For this review, take the finished solid that the model builds, in its own axes (mm). Give positions to 0.01 mm unless a question says otherwise; leave off trailing zeros. Order: outer loops, then holes, each group sorted by start corner. A loop starts at its lowest first (then second) coordinate and runs counter-clockwise, first axis right, second up.
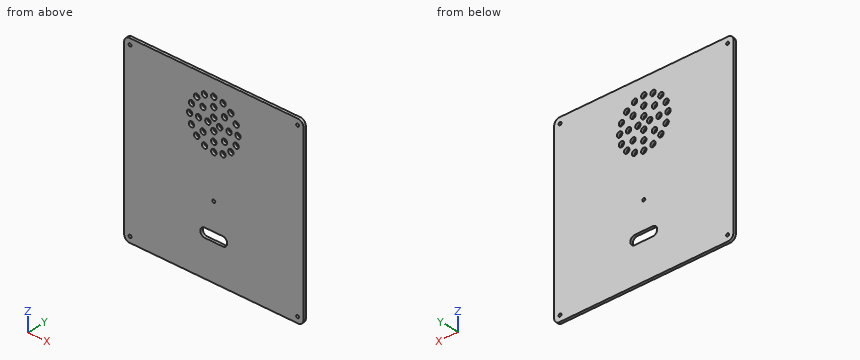
from build123d import *

# Parameters (mm, degrees)
SKETCH1_W           = 200
SKETCH1_H           = 200
SKETCH1_R           = 3
BOSS_EXTRUDE1_DEPTH = 3
FILLET1_R           = 6
FILLET2_R           = 6
FILLET3_R           = 6
FILLET4_R           = 6
SKETCH2_R           = 1.65
SKETCH2_R_2         = 5
CUT_EXTRUDE1_DEPTH  = 283.85862193


with BuildPart() as part:
    # Sketch1 → Boss-Extrude1 (new body)
    with BuildSketch(Plane(origin=(0, 0, 0), x_dir=(1, 0, 0), z_dir=(0, 1, 0))):
        with Locations((100, 100)):
            Rectangle(SKETCH1_W, SKETCH1_H)
        with Locations(Location((116.974857902, 45, 0), (0, 0, 270))):
            Circle(SKETCH1_R, mode=Mode.SUBTRACT)
        with Locations(Location((112.003037132, 32.996962868, 0), (0, 0, 270))):
            Circle(SKETCH1_R, mode=Mode.SUBTRACT)
        with Locations(Location((100, 28.025142098, 0), (0, 0, 270))):
            Circle(SKETCH1_R, mode=Mode.SUBTRACT)
        with Locations(Location((87.996962868, 32.996962868, 0), (0, 0, 270))):
            Circle(SKETCH1_R, mode=Mode.SUBTRACT)
        with Locations(Location((83.025142098, 45, 0), (0, 0, 270))):
            Circle(SKETCH1_R, mode=Mode.SUBTRACT)
        with Locations(Location((87.996962868, 57.003037132, 0), (0, 0, 270))):
            Circle(SKETCH1_R, mode=Mode.SUBTRACT)
        with Locations(Location((100, 61.974857902, 0), (0, 0, 270))):
            Circle(SKETCH1_R, mode=Mode.SUBTRACT)
        with Locations(Location((112.003037132, 57.003037132, 0), (0, 0, 270))):
            Circle(SKETCH1_R, mode=Mode.SUBTRACT)
        with Locations(Location((126.974857902, 45, 0), (0, 0, 270))):
            Circle(SKETCH1_R, mode=Mode.SUBTRACT)
        with Locations(Location((124.921888894, 34.679027829, 0), (0, 0, 270))):
            Circle(SKETCH1_R, mode=Mode.SUBTRACT)
        with Locations(Location((119.075527791, 25.929330111, 0), (0, 0, 270))):
            Circle(SKETCH1_R, mode=Mode.SUBTRACT)
        with Locations(Location((110.325830073, 20.082969008, 0), (0, 0, 270))):
            Circle(SKETCH1_R, mode=Mode.SUBTRACT)
        with Locations(Location((100.004857902, 18.03, 0), (0, 0, 270))):
            Circle(SKETCH1_R, mode=Mode.SUBTRACT)
        with Locations(Location((89.683885731, 20.082969008, 0), (0, 0, 270))):
            Circle(SKETCH1_R, mode=Mode.SUBTRACT)
        with Locations(Location((80.934188014, 25.929330111, 0), (0, 0, 270))):
            Circle(SKETCH1_R, mode=Mode.SUBTRACT)
        with Locations(Location((75.08782691, 34.679027829, 0), (0, 0, 270))):
            Circle(SKETCH1_R, mode=Mode.SUBTRACT)
        with Locations(Location((106.559618743, 45, 0), (0, 0, 270))):
            Circle(SKETCH1_R, mode=Mode.SUBTRACT)
        with Locations(Location((100, 38.440381257, 0), (0, 0, 270))):
            Circle(SKETCH1_R, mode=Mode.SUBTRACT)
        with Locations(Location((93.440381257, 45, 0), (0, 0, 270))):
            Circle(SKETCH1_R, mode=Mode.SUBTRACT)
        with Locations(Location((100, 51.559618743, 0), (0, 0, 270))):
            Circle(SKETCH1_R, mode=Mode.SUBTRACT)
        with Locations(Location((73.034857902, 45, 0), (0, 0, 270))):
            Circle(SKETCH1_R, mode=Mode.SUBTRACT)
        with Locations(Location((75.08782691, 55.320972171, 0), (0, 0, 270))):
            Circle(SKETCH1_R, mode=Mode.SUBTRACT)
        with Locations(Location((80.934188014, 64.070669889, 0), (0, 0, 270))):
            Circle(SKETCH1_R, mode=Mode.SUBTRACT)
        with Locations(Location((89.683885731, 69.917030992, 0), (0, 0, 270))):
            Circle(SKETCH1_R, mode=Mode.SUBTRACT)
        with Locations(Location((100.004857902, 71.97, 0), (0, 0, 270))):
            Circle(SKETCH1_R, mode=Mode.SUBTRACT)
        with Locations(Location((110.325830073, 69.917030992, 0), (0, 0, 270))):
            Circle(SKETCH1_R, mode=Mode.SUBTRACT)
        with Locations(Location((119.075527791, 64.070669889, 0), (0, 0, 270))):
            Circle(SKETCH1_R, mode=Mode.SUBTRACT)
        with Locations(Location((124.921888894, 55.320972171, 0), (0, 0, 270))):
            Circle(SKETCH1_R, mode=Mode.SUBTRACT)
    extrude(amount=BOSS_EXTRUDE1_DEPTH)

    # Fillet1
    fillet1_edges = [part.edges().sort_by_distance(p)[0] for p in [
        (0, 1.5, -200),
    ]]
    fillet(fillet1_edges, radius=FILLET1_R)

    # Fillet2
    fillet2_edges = [part.edges().sort_by_distance(p)[0] for p in [
        (200, 1.5, -200),
    ]]
    fillet(fillet2_edges, radius=FILLET2_R)

    # Fillet3
    fillet3_edges = [part.edges().sort_by_distance(p)[0] for p in [
        (200, 1.5, 0),
    ]]
    fillet(fillet3_edges, radius=FILLET3_R)

    # Fillet4
    fillet4_edges = [part.edges().sort_by_distance(p)[0] for p in [
        (0, 1.5, 0),
    ]]
    fillet(fillet4_edges, radius=FILLET4_R)

    # Sketch2 → Cut-Extrude1 (cut, through all)
    with BuildSketch(Plane(origin=(0, 3, 0), x_dir=(1, 0, 0), z_dir=(0, 1, 0))):
        with Locations(Location((6.5, 6.5, 0), (0, 0, 270))):
            Circle(SKETCH2_R)
        with Locations(Location((193.5, 6.5, 0), (0, 0, 270))):
            Circle(SKETCH2_R)
        with Locations(Location((193.5, 193.5, 0), (0, 0, 270))):
            Circle(SKETCH2_R)
        with Locations((90, 155)):
            Circle(SKETCH2_R_2)
        with BuildLine():
            ThreePointArc((110, 150), (105, 155), (110, 160))
            Line((110, 160), (90, 160))
            ThreePointArc((90, 160), (93.535533906, 158.535533906), (95, 155))
            ThreePointArc((95, 155), (93.535533906, 151.464466094), (90, 150))
            Line((90, 150), (110, 150))
        make_face()
        with Locations((110, 155)):
            Circle(SKETCH2_R_2)
        with Locations(Location((100, 120, 0), (0, 0, 270))):
            Circle(SKETCH2_R)
        with Locations(Location((6.5, 193.5, 0), (0, 0, 270))):
            Circle(SKETCH2_R)
    extrude(amount=-CUT_EXTRUDE1_DEPTH, mode=Mode.SUBTRACT)


solid = part.part
1) We need section C-C on y = 2.5. Count the separate pieces of the cut face and the enclosed holes in it, then the cut area to 3 significant figures.
Answer sheet:
separate pieces: 1
enclosed holes: 34
area: 38,900 mm2
2) We need section B-B on z = -45. Give the boundary of the cut face in (x, y), then the cut area to 3 significant figures.
Answer sheet:
outline: (0, 0) - (70.03, 0) - (70.03, 3) - (0, 3) - close; (76.03, 0) - (80.03, 0) - (80.03, 3) - (76.03, 3) - close; (86.03, 0) - (90.44, 0) - (90.44, 3) - (86.03, 3) - close; (96.44, 0) - (103.56, 0) - (103.56, 3) - (96.44, 3) - close; (109.56, 0) - (113.97, 0) - (113.97, 3) - (109.56, 3) - close; (119.97, 0) - (123.97, 0) - (123.97, 3) - (119.97, 3) - close; (129.97, 0) - (200, 0) - (200, 3) - (129.97, 3) - close
area: 492 mm2
3) We need section A-A on z = -155. Give the boundary of the cut face in (x, y), then the cut area to 3 significant figures.
Answer sheet:
outline: (0, 0) - (85, 0) - (85, 3) - (0, 3) - close; (115, 0) - (200, 0) - (200, 3) - (115, 3) - close
area: 510 mm2
4) To check wall thickness, follow line 1 (X direction, y = 1.05, z = -6.5); line 2 (Z direction, x = 116.5, y = 2.8); line 3 (X direction, y = 1.55, z = -57). State the ranges of each line that lie inside material, in increasing order.
Answer sheet:
line 1: x = 0 to 4.85, 8.15 to 191.85, 195.15 to 200
line 2: z = -200 to -65.61, -62.53 to -47.96, -42.04 to -27.47, -24.39 to 0
line 3: x = 0 to 72.6, 77.57 to 85, 91 to 109, 115 to 122.44, 127.41 to 200
